The model under review builds one solid part; all positions refer to its coordinate system, in mm. A direction names the side the tool comes from. Round coordinates to 2 decimals unless told otherwise and drop trailing zeros. Write each loop counter-clockwise with the first axis right and the second up, starting at its lowest first coordinate (ties: lowest second). Pieces come first, ordered by that corner, then holes. Notation, with made-up numbers: (48.5, 38) -> (54.5, 38) arc R8 ccw to (54.5, 53) -> close; hole circle Ø1 at (-35, -30.75). An arc over 180 degrees is marked (long way). Use CSV: the item, a comma, the result in double quotes. Start each with the question number.
1) Take a section at D-D, the plane y = -363. Give the boundary of the cut face in (x, z) (3 decimals).
2) Take a section at C-C, the plane x = 5. Give the boundary of the cut face in (y, z).
3) Take a section at B-B, the plane y = -178. Give the boundary of the cut face in (x, z) (3 decimals).
4) For pin 1 Ø1.5 at (x, z) = (-19.5, -20) entering from +Y; pin 2 Ø12 at (x, z) = (7.5, 28.5) entering from +Y, all flat-tipped, find the tip position at first contact; note any pin that passes through.
5) Mouldability with a two-part tool opening along X and no side actions: class faces 1 (the face through (-19.05, -200, 0)), 2 (the face through (-22.54, -200.36, 35.38)), 3 (the face through (-22.2, -367.8, -0.5)) as released by +X, released by -X, zero draft, split by the parting line, or undercut.
6) Machinability: for faces 4 (the face through (19.05, -200, 0)), 5 (the face through (22.68, -200.36, 35.24)), which of the approach directions +Z, -Z, +X, -X, +Y, -Y give a long, thin tool a straight path to every point of the face, cutting with its end or side? Answer none if there is none.
7) Take a section at A-A, the plane z = 9. Give the boundary of the cut face in (x, y), then the cut area to 3 significant figures.
8) Wall thickness on probe 1 along Z at (x, y) = (-5, -165.5); probe 2 along X at (y, z) = (-242.5, 13.5); probe 3 along Z at (x, y) = (15, -342): over which ranges is each line inside the solid? List them lowest first. Write a range as [from, to].
from build123d import *

# Parameters (mm, degrees)
F1_DEPTH = 406.4
F3_DEPTH = 50.8


with BuildPart() as f1:
    # F0 (on Front) → F1 (new body)
    with BuildSketch(Plane.XZ):
        with BuildLine():
            ThreePointArc((-25.4, -28.575), (-22.6101920908, -35.3101920908), (-15.875, -38.1))
            Line((-15.875, -38.1), (15.875, -38.1))
            ThreePointArc((15.875, -38.1), (22.6101920908, -35.3101920908), (25.4, -28.575))
            Line((25.4, -28.575), (25.4, 28.575))
            ThreePointArc((25.4, 28.575), (22.6101920908, 35.3101920908), (15.875, 38.1))
            Line((15.875, 38.1), (-15.875, 38.1))
            ThreePointArc((-15.875, 38.1), (-22.6101920908, 35.3101920908), (-25.4, 28.575))
            Line((-25.4, 28.575), (-25.4, -28.575))
        make_face()
        with BuildLine():
            ThreePointArc((19.0500010133, -28.575), (18.1200647468, -30.8200647468), (15.875, -31.7500010133))
            Line((15.875, -31.7500010133), (-15.875, -31.7500010133))
            ThreePointArc((-15.875, -31.7500010133), (-18.1200647468, -30.8200647468), (-19.0500010133, -28.575))
            Line((-19.0500010133, -28.575), (-19.0500010133, 28.575))
            ThreePointArc((-19.0500010133, 28.575), (-18.1200647468, 30.8200647468), (-15.875, 31.7500010133))
            Line((-15.875, 31.7500010133), (15.875, 31.7500010133))
            ThreePointArc((15.875, 31.7500010133), (18.1200647468, 30.8200647468), (19.0500010133, 28.575))
            Line((19.0500010133, 28.575), (19.0500010133, -28.575))
        make_face(mode=Mode.SUBTRACT)
    extrude(amount=F1_DEPTH)

    # F2 (on Right) → F3 (cut, symmetric)
    with BuildSketch(Plane.YZ):
        Polygon((0, -38.1), (0, 38.1), (-76.2, -38.1), align=None)
        Polygon((-330.2, -38.1), (-406.4, 38.1), (-406.4, -38.1), align=None)
    extrude(amount=F3_DEPTH, both=True, mode=Mode.SUBTRACT)


with BuildPart() as f4_1:
    # F4: copy of F1
    add(f1.part)


solid = f1.part
Values found:
1,outline,"(-25.4, -5.3) -> (-19.05, -5.3) -> (-19.05, 28.575) arc R3.175 cw to (-15.875, 31.75) -> (15.875, 31.75) arc R3.175 cw to (19.05, 28.575) -> (19.05, -5.3) -> (25.4, -5.3) -> (25.4, 28.575) arc R9.525 ccw to (15.875, 38.1) -> (-15.875, 38.1) arc R9.525 ccw to (-25.4, 28.575) -> close"
2,outline,"(-406.4, 38.1) -> (-400.05, 31.75) -> (-6.35, 31.75) -> (0, 38.1) -> close; (-336.55, -31.75) -> (-330.2, -38.1) -> (-76.2, -38.1) -> (-69.85, -31.75) -> close"
3,outline,"(-25.4, -28.575) arc R9.525 ccw to (-15.875, -38.1) -> (15.875, -38.1) arc R9.525 ccw to (25.4, -28.575) -> (25.4, 28.575) arc R9.525 ccw to (15.875, 38.1) -> (-15.875, 38.1) arc R9.525 ccw to (-25.4, 28.575) -> close; hole (-19.05, -28.575) arc R3.175 ccw to (-15.875, -31.75) -> (15.875, -31.75) arc R3.175 ccw to (19.05, -28.575) -> (19.05, 28.575) arc R3.175 ccw to (15.875, 31.75) -> (-15.875, 31.75) arc R3.175 ccw to (-19.05, 28.575) -> close"
4,pin 1,"y = -57.35"
4,pin 2,"y = -3.6"
5,face 1,"undercut"
5,face 2,"released by -X"
5,face 3,"zero draft"
6,face 4,"+Y, -Y"
6,face 5,"+Z, +X, +Y, -Y"
7,outline,"(-25.4, -377.3) -> (-19.05, -377.3) -> (-19.05, -29.1) -> (-25.4, -29.1) -> close; (19.05, -377.3) -> (25.4, -377.3) -> (25.4, -29.1) -> (19.05, -29.1) -> close"
7,area,"4,420 mm²"
8,probe 1,"[-38.1, -31.75], [31.75, 38.1]"
8,probe 2,"[-25.4, -19.05], [19.05, 25.4]"
8,probe 3,"[31.75, 38.1]"
